The model under review builds one solid part; all positions refer to its coordinate system, in mm. Coordinates: 2 decimals unless noted, no trailing zeros. Loops run counter-clockwise (first coordinate to the right, second up) from the corner with the lowest first, then second, coordinate; pieces in that order, holes last. Notation, with made-up numbers: M 88.25,-34 L 97.25,-34 A21 cw 97.25,-20 Z; hole C 50,77 d9. An arc over 180 degrees is marked long. Use CSV: the item, a comma, the result in double quotes. Start each with the question number.
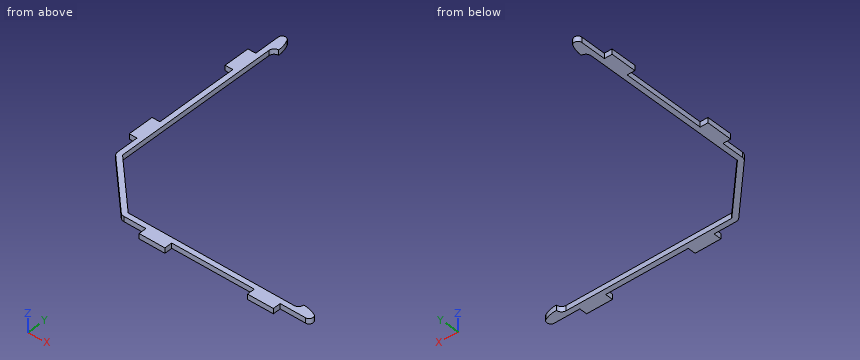
Autodesk Fusion 360 part; units mm, degrees
sketch "Sketch1" plane through (0, 0, 0) normal (0, 0, 1) x (1, 0, 0)
  line L0 (-60.9778, -51.3602) -> (-51.369, -60.969)
  arc A0 (-51.369, -60.969) -> (-50.57, -61.3) centre (-50.57, -60.17) ccw
  line L1 (-50.8444, -61.3) -> (-15.6217, -61.3)
  arc A1 (-15.2933, -59.8758) -> (-17.7897, -59.3) centre (-17.7897, -65) ccw
  arc A2 (-18.7897, -60.3) -> (-17.7897, -59.3) centre (-18.7897, -59.3) ccw
  line L2 (-18.7897, -60.3) -> (-50.8444, -60.3)
  arc A3 (-50.6619, -60.2619) -> (-50.57, -60.3) centre (-50.57, -60.17) ccw
  line L3 (-50.6619, -60.2619) -> (-60.2707, -50.6531)
  arc A4 (-60.3, -50.5824) -> (-60.2707, -50.6531) centre (-60.2, -50.5824) ccw
  line L4 (-60.3, -50.8444) -> (-60.3, -18.8024)
  arc A5 (-59.3, -17.8024) -> (-60.3, -18.8024) centre (-59.3, -18.8024) ccw
  arc A6 (-59.3, -17.8024) -> (-59.8758, -15.306) centre (-65, -17.8024) ccw
  line L5 (-61.3, -15.6345) -> (-61.3, -50.8444)
  arc A7 (-61.3, -50.5824) -> (-60.9778, -51.3602) centre (-60.2, -50.5824) ccw
  arc A8 (-15.6217, -61.3) -> (-15.2933, -59.8758) centre (-15.6217, -60.55) ccw
  arc A9 (-59.8758, -15.306) -> (-61.3, -15.6345) centre (-60.55, -15.6345) ccw
  line L6 (-62.8, -15.6345) -> (-62.8, -50.8444)
  line L7 (-50.8444, -62.8) -> (-15.6217, -62.8)
  line L8 (-61.3, -46.5824) -> (-62.8, -46.5824)
  line L9 (-62.8, -41.5824) -> (-61.3, -41.5824)
  line L10 (-62.8, -20.5824) -> (-61.3, -20.5824)
  line L11 (-62.8, -25.5824) -> (-61.3, -25.5824)
  line L12 (-46.57, -61.3) -> (-46.57, -62.8)
  line L13 (-41.57, -61.3) -> (-41.57, -62.8)
  line L14 (-25.57, -61.3) -> (-25.57, -62.8)
  line L15 (-20.57, -61.3) -> (-20.57, -62.8)
  arc A10 (-51.6222, -60.9778) -> (-50.8444, -61.3) centre (-50.8444, -60.2) ccw
  line L16 (-60.9778, -51.6222) -> (-51.6222, -60.9778)
  arc A11 (-61.3, -50.8444) -> (-60.9778, -51.6222) centre (-60.2, -50.8444) ccw
  arc A12 (-60.3, -50.8444) -> (-60.2707, -50.9151) centre (-60.2, -50.8444) ccw
  line L17 (-50.9151, -60.2707) -> (-60.2707, -50.9151)
  arc A13 (-50.9151, -60.2707) -> (-50.8444, -60.3) centre (-50.8444, -60.2) ccw
  dimension "d1" = 60.3
  dimension "d2" = 60.3
  dimension "d3" = 1
  dimension "d4" = 1
  dimension "d5" = 1
  dimension "d6" = 5.7
  dimension "d7" = 0.75
  dimension "d8" = 3.7
  dimension "d9" = 1.13
  dimension "d10" = 1.1
  dimension "d11" = 45
  dimension "d12" = 50.57
  dimension "d13" = 31.7803
  dimension "d14" = 1
  dimension "d15" = 31.78
  dimension "d16" = 1
  dimension "d17" = 5.7
  dimension "d18" = 3.7
  dimension "d19" = 1
  dimension "d21" = 0.75
  dimension "d22" = 1.5
  dimension "d23" = 1.5
  dimension "d24" = 4
  dimension "d25" = 4
  dimension "d26" = 5
  dimension "d27" = 5
  dimension "d28" = 16
  dimension "d29" = 5
  dimension "d30" = 16
  dimension "d31" = 5
extrude "Extrude1" add sketch "Sketch1" along normal blind 1 contours L0 A0 L1 A1 A2 L2 L4 A5 A6 L5 A7 A8 A9 A12 L17 A13 | L0 A0 L1 L5 A7 A10 L16 A11 | L5 L6 L8 L9 | L1 L7 L12 L13 | L5 L6 L10 L11 | L1 L7 L14 L15
1. Add section C-C (y = -37). Write out the cut boundary in (x, z), plus the area to 3 significant figures.
2. Insertion check: pin 1 Ø0.5 at (y, z) = (-37, 0.5) entering from -X; pin 2 Ø10 at (x, y) = (-47, -54.5) entering from +Z; pin 3 Ø0.5 at (x, z) = (-17.5, 0.5) entering from -Y. Each pin has a flat end and moves straight along its axis. Give the tip position at first contact, or say it passes through.
3. To check wall thickness, follow line 1 along Y through (x, z) = (-38, 0.45); line 2 along Y through (x, z) = (-22, 0.5). State the ranges of each line that lie inside material, in increasing order.
4. Add section B-B (x = -44). Write out the cut boundary in (y, z).
Solved:
1,outline,"M -61.3,0 L -60.3,0 L -60.3,1 L -61.3,1 Z"
1,area,"1.00 mm^2"
2,pin 1,"stops at x = -61.3"
2,pin 2,"passes through"
2,pin 3,"stops at y = -61.3"
3,line 1,"y = -61.3 to -60.3"
3,line 2,"y = -62.8 to -60.3"
4,outline,"M -62.8,0 L -60.3,0 L -60.3,1 L -62.8,1 Z"
